Geometry: final body of the model. Coordinates: model frame, mm. Face numbers are marked on the shaded views. A direction names the side the tool comes from. Give positions to 0.01 mm unless a question says otherwise; leave off trailing zeros. Write each loop counter-clockwise with the first axis right and the second up, starting at its lowest first coordinate (ties: lowest second). Pieces come first, ordered by that corner, then holes.
Q1. Cut plane A-A on z = 13. Return the cut outline in (x, y).
Q2. Cut plane D-D on x = -4.5. Return the cut outline in (y, z), plus the area to 3 significant figures.
Q3. Draft query along X for the marked faces 1, 2 and 3. Return one class per face: pulls with the +X half, pulls with the -X half, needs draft (parallel to the pull), parting line crosses it, or undercut.
Q4. Reachability of the marked faces 4, 5 and 6 from +Z, -Z, +X, -X, +Y, -Y: full face, straight path, thin tool, end or side. Return the list, or none.
Q5. Pin query (flat end, axial travel): pin 1 (5 mm diameter, centred on x = -4.5, y = 7, fed in from +Z); pin 2 (4.5 mm diameter, centred on x = -5.5, y = 4, fed in from -Z); pin 3 (0.6 mm diameter, centred on x = 1, y = -3.5, fed in from -Z); pin 4 (4 mm diameter, centred on x = 5, y = -5.5, fed in from +Z). Return the tip coordinate at first contact, or that it passes through.
Q6. Cut plane B-B on y = 1.5. Return the cut outline in (x, z).
Q7. Cut plane C-C on x = 7. Return the cut outline in (y, z), plus the area to 3 significant figures.
Q8. Line query: L1, parallel to Y at x = 0.25, z = 9.75; L2, parallel to X at y = 0, z = 15.75; L3, parallel to Y at x = -0.25, z = 24.5. Output: solid intervals per line, ascending.
```python
from build123d import *

# Parameters (mm, degrees)
CYLINDER021_R     = 5
CYLINDER021_DEPTH = 25
CYLINDER022_R     = 5
CYLINDER022_DEPTH = 15
CYLINDER020_R     = 9
CYLINDER020_DEPTH = 9.5
BOX007_W          = 19
BOX007_H          = 18
BOX007_DEPTH      = 19.5
FILLET_R          = 8.5


with BuildPart() as obj1_hole:
    # Cylinder021 → Cylinder021 (new body)
    with BuildSketch(Plane.XY):
        Circle(CYLINDER021_R)
    extrude(amount=CYLINDER021_DEPTH)


with BuildPart() as obj2:
    # Cylinder022 → Cylinder022 (new body)
    with BuildSketch(Plane(origin=(-5, 0, 21), x_dir=(0, 0, -1), z_dir=(1, 0, 0))):
        Circle(CYLINDER022_R)
    extrude(amount=CYLINDER022_DEPTH)

    # Fusion016: union obj1_hole
    add(obj1_hole.part)


with BuildPart() as obj1:
    # Cylinder020 → Cylinder020 (new body)
    with BuildSketch(Plane.XY):
        Circle(CYLINDER020_R)
    extrude(amount=CYLINDER020_DEPTH)


with BuildPart() as obj3:
    # Box007 → Box007 (new body)
    with BuildSketch(Plane(origin=(-9, -9, 9.5), x_dir=(1, 0, 0), z_dir=(0, 0, 1))):
        with Locations((9.5, 9)):
            Rectangle(BOX007_W, BOX007_H)
    extrude(amount=BOX007_DEPTH)

    # Fillet
    fillet_edges = [obj3.edges().sort_by_distance(p)[0] for p in [
        (-9, -9, 19.25),
        (-9, 0, 29),
        (-9, 9, 19.25),
        (0.5, -9, 29),
        (0.5, 9, 29),
    ]]
    fillet(fillet_edges, radius=FILLET_R)

    # Fusion018: union obj1
    add(obj1.part)

    # Cut009: cut obj2
    add(obj2.part, mode=Mode.SUBTRACT)


solid = obj3.part
```
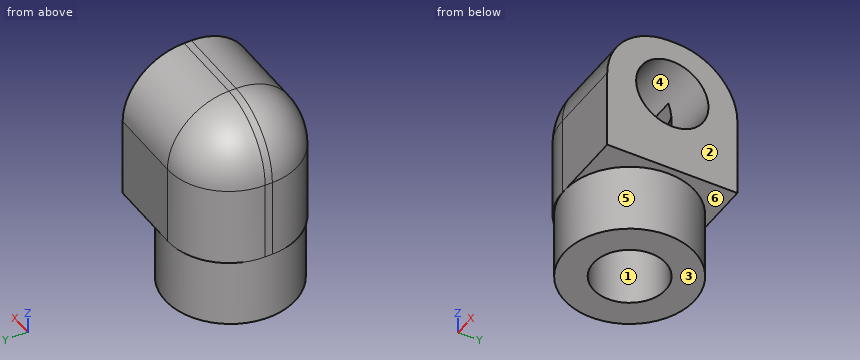
Data:
1. outline: (-9, -0.5) arc R8.5 ccw to (-0.5, -9) - (10, -9) - (10, 9) - (-0.5, 9) arc R8.5 ccw to (-9, 0.5) - close; hole circle Ø10 at (0, 0)
2. outline: (-8, 9.5) - (-7.79, 9.5) - (-7.79, 0) - (-2.18, 0) - (-2.18, 16.5) arc R5 cw (long way) to (2.18, 16.5) - (2.18, 0) - (7.79, 0) - (7.79, 9.5) - (8, 9.5) - (8, 20.5) arc R7.5 ccw to (0.5, 28) - (-0.5, 28) arc R7.5 ccw to (-8, 20.5) - close
2. area: 271 mm2
3. face 1: undercut
3. face 2: pulls with the +X half
3. face 3: needs draft
4. face 4: +X
4. face 5: -Z
4. face 6: -Z, +X
5. pin 1: stops at z = 27.28
5. pin 2: stops at z = 0
5. pin 3: stops at z = 25
5. pin 4: stops at z = 28.45
6. outline: (-8.94, 9.5) - (-8.87, 9.5) - (-8.87, 0) - (-4.77, 0) - (-4.77, 16.23) - (-5, 16.23) - (-5, 25.77) - (10, 25.77) - (10, 28.94) - (-0.5, 28.94) arc R8.44 ccw to (-8.94, 20.5) - close; (4.77, 0) - (8.87, 0) - (8.87, 9.5) - (10, 9.5) - (10, 16.23) - (4.77, 16.23) - close
7. outline: (-9, 9.5) - (-5.66, 9.5) - (-5.66, 0) - (5.66, 0) - (5.66, 9.5) - (9, 9.5) - (9, 20.5) arc R8.5 ccw to (0.5, 29) - (-0.5, 29) arc R8.5 ccw to (-9, 20.5) - close; hole circle Ø10 at (0, 21)
7. area: 349 mm2
8. L1: y = -9 to -4.99, 4.99 to 9
8. L2: x = -9 to -5, 5 to 10
8. L3: y = -8 to -4.99, 4.99 to 8
